from build123d import *

# Parameters (mm, degrees)
SKETCH_1_R          = 8
EXTRUDE_1_DEPTH     = 75.5
CHAMFER_1_SIZE      = 0.5
SKETCH_3_R          = 4
CUT_EXTRUDE_1_DEPTH = 23
SKETCH_4_R          = 2
CUT_EXTRUDE_2_DEPTH = 23


with BuildPart() as part:
    # 스케치1 → 보스-돌출1 (new body)
    with BuildSketch(Plane(origin=(0, 0, 0), x_dir=(1, 0, 0), z_dir=(0, 1, 0))):
        with Locations(Location((0, 0, 0), (0, 0, 270))):
            Circle(SKETCH_1_R)
    extrude(amount=-EXTRUDE_1_DEPTH)

    # 모따기1
    chamfer_1_edges = [part.edges().sort_by_distance(p)[0] for p in [
        (0, 0, -8),
    ]]
    chamfer(chamfer_1_edges, length=CHAMFER_1_SIZE)

    # 스케치3 → 컷-돌출1 (cut)
    with BuildSketch(Plane(origin=(0, 0, 0), x_dir=(1, 0, 0), z_dir=(0, 1, 0))):
        with Locations(Location((0, 0, 0), (0, 0, 270))):
            Circle(SKETCH_3_R)
    extrude(amount=-CUT_EXTRUDE_1_DEPTH, mode=Mode.SUBTRACT)

    # 스케치4 → 컷-돌출2 (cut)
    with BuildSketch(Plane(origin=(0, 0, 0), x_dir=(0, 0, -1), z_dir=(1, 0, 0))):
        with Locations((0, -5)):
            Circle(SKETCH_4_R)
    extrude(amount=-CUT_EXTRUDE_2_DEPTH, mode=Mode.SUBTRACT)


solid = part.part
Here's how the part is built. I have some questions about the finished solid (model axes, mm). A direction names the side the tool comes from. Coordinates: 2 decimals unless noted, no trailing zeros. Order: outer loops, then holes, each group sorted by start corner. A loop starts at its lowest first (then second) coordinate and runs counter-clockwise, first axis right, second up.
Item 1: For P1, Ø8, axis at x = -6, y = -20.5, coming from the -Z side; P2, Ø7, axis at x = 0, z = 0, coming from the +Y side; P3, Ø2, axis at y = -51, z = -3.5, coming from the +X side; P4, Ø2, axis at x = 1, y = -45, coming from the -Z side, each with a flat end and sliding along its axis, tell me the tip position at first contact or that it passes through.
Result sheet:
P1: stops at z = -7.75
P2: stops at y = -23
P3: stops at x = 7.6
P4: stops at z = -8
Item 2: If we mould it in two halves opening along Z, with no side actions, what happens to faces 3 (the face through (-3, 0, 3)), 4 (the face through (-6, -7, 0)), 5 (the face through (0, -23, 0)), 6 (the face through (7.932, -37.475, -1.041))? For each: +Z half, -Z half, draft (parallel to the pull), parting line (faces both ways), or undercut.
Result sheet:
face 3: draft
face 4: undercut
face 5: undercut
face 6: parting line
Item 3: For faces 1 (the face through (3.966, -11.339, -0.521)), 2 (the face through (0, -75.5, 0)), which set-ups out of +Z, -Z, +X, -X, +Y, -Y let a thin tool reach every point of the face, with its end or its side?
Result sheet:
face 1: +Y
face 2: +Z, -Z, +X, -X, -Y
Item 4: I need wall thicknesses on line 1 (Y direction, x = -6.4, z = 0); line 2 (X direction, y = -15, z = 0); line 3 (Z direction, x = 0.25, y = -67.5). Which ranges of each line are inside material? Lowest first, please.
Result sheet:
line 1: y = -75.5 to -7, -3 to 0
line 2: x = -8 to -4, 4 to 8
line 3: z = -8 to 8
Item 5: If we section it at D-D on y = -56: List the corners of the cut face in (x, z) for me, plus the area to 3 significant figures.
Result sheet:
outline: circle Ø16 at (0, 0)
area: 201 mm2
Item 6: If we section it at B-B on x = 0: List the corners of the cut face in (y, z) for me, plus the area to 3 significant figures.
Result sheet:
outline: (-75.5, -8) - (-0.5, -8) - (0, -7.5) - (0, -4) - (-23, -4) - (-23, 4) - (0, 4) - (0, 7.5) - (-0.5, 8) - (-75.5, 8) - close
area: 1,020 mm2
Item 7: If we section it at A-A on z = 0: List the corners of the cut face in (x, y) for me, plus the area to 3 significant figures.
Result sheet:
outline: (-8, -75.5) - (8, -75.5) - (8, -0.5) - (7.5, 0) - (4, 0) - (4, -23) - (-4, -23) - (-4, -7) - (-8, -7) - close; (-8, -3) - (-4, -3) - (-4, 0) - (-7.5, 0) - (-8, -0.5) - close
area: 1,010 mm2
Item 8: If we section it at C-C on y = -16: List the corners of the cut face in (x, z) for me.
Result sheet:
outline: circle Ø16 at (0, 0); hole circle Ø8 at (0, 0)
